Build history of the part. All positions in model axes, mm. Face numbers are marked on the shaded views. A direction names the side the tool comes from. Coordinates: 2 decimals unless noted, no trailing zeros. Loops run counter-clockwise (first coordinate to the right, second up) from the corner with the lowest first, then second, coordinate; pieces in that order, holes last. Notation, with made-up numbers: (67.25, -11.5) - (115.25, -11.5) arc R5 cw to (115.25, -4.5) - close; hole circle Ø8 at (71, 41). An arc over 180 degrees is marked (long way). One line per item, written item: value.
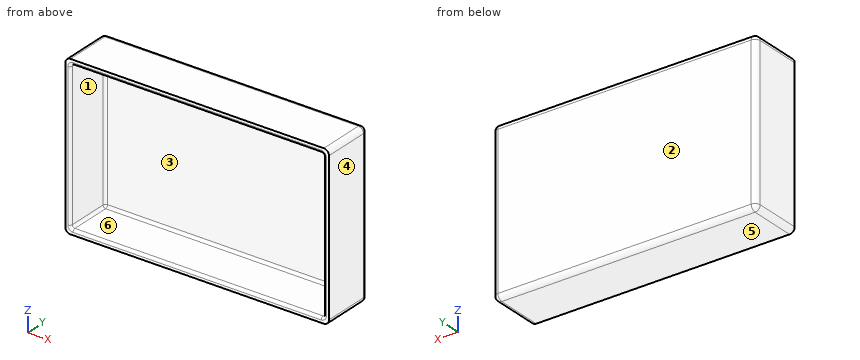
```python
from build123d import *

# Parameters (mm, degrees)
BOSS_EXTRUDE1_DEPTH = 20
FILLET1_R           = 2
SHELL1_START        = -49
SHELL1_OUTLINE_W    = 18
SHELL1_OUTLINE_H    = 58
SHELL1_DEPTH        = 98
FILLET2_R           = 1


# Read off the part's stored shape, not the designer's step: Shell1
with BuildPart() as part:
    # Sketch1 → Boss-Extrude1 (new body)
    with BuildSketch(Plane(origin=(0, 0, 0), x_dir=(1, 0, 0), z_dir=(0, 1, 0))):
        with BuildLine():
            Line((-49, -31), (49, -31))
            ThreePointArc((49, -31), (50.414213562, -30.414213562), (51, -29))
            Line((51, -29), (51, 29))
            ThreePointArc((51, 29), (50.414213562, 30.414213562), (49, 31))
            Line((49, 31), (-49, 31))
            ThreePointArc((-49, 31), (-50.414213562, 30.414213562), (-51, 29))
            Line((-51, 29), (-51, -29))
            ThreePointArc((-51, -29), (-50.414213562, -30.414213562), (-49, -31))
        make_face()
    extrude(amount=BOSS_EXTRUDE1_DEPTH)

    # Fillet1
    fillet1_edges = [part.edges().sort_by_distance(p)[0] for p in [
        (50.414213562, 20, -30.414213562),
        (0, 20, -31),
        (-50.414213562, 20, -30.414213562),
        (-51, 20, 0),
        (-50.414213562, 20, 30.414213562),
        (0, 20, 31),
        (50.414213562, 20, 30.414213562),
        (51, 20, 0),
    ]]
    fillet(fillet1_edges, radius=FILLET1_R)

    # Shell1 outline → Shell1 (cut)
    with BuildSketch(Plane.YZ.offset(SHELL1_START)):
        with Locations((9, 0)):
            Rectangle(SHELL1_OUTLINE_W, SHELL1_OUTLINE_H)
    extrude(amount=SHELL1_DEPTH, mode=Mode.SUBTRACT)

    # Fillet2
    fillet2_edges = [part.edges().sort_by_distance(p)[0] for p in [
        (49, 9, 29),
        (49, 0, 0),
        (0, 18, -29),
        (49, 9, -29),
        (0, 0, -29),
        (-49, 18, 0),
        (-49, 9, -29),
        (-49, 0, 0),
        (0, 18, 29),
        (-49, 9, 29),
        (0, 0, 29),
        (49, 18, 0),
    ]]
    fillet(fillet2_edges, radius=FILLET2_R)


solid = part.part
```
Item 1: Cut at A-A, the plane y = 13.5. Write the cut outline in (x, z).
Check result:
outline: (-51, -29) arc R2 ccw to (-49, -31) - (49, -31) arc R2 ccw to (51, -29) - (51, 29) arc R2 ccw to (49, 31) - (-49, 31) arc R2 ccw to (-51, 29) - close; hole (-49, -28) arc R1 ccw to (-48, -29) - (48, -29) arc R1 ccw to (49, -28) - (49, 28) arc R1 ccw to (48, 29) - (-48, 29) arc R1 ccw to (-49, 28) - close
Item 2: Tool access for the marked faces 1 and 2: list every direction of +Z, -Z, +X, -X, +Y, -Y with a clear straight run to the whole face (end or side of a thin tool).
Check result:
face 1: -Y
face 2: +Z, -Z, +X, -X, +Y
Item 3: Drop a flat-ended pin along its axis: P1, Ø2, axis at x = 3, z = 23, coming from the -Y side. Give the stop position or say it passes through.
Check result:
P1: stops at y = 18
Item 4: Pull direction X, two halves, no side cores. Call the marked faces 3, 4, 5 and 6: released by +X, released by -X, zero draft, split by the parting line, or undercut.
Check result:
face 3: undercut
face 4: released by +X
face 5: zero draft
face 6: undercut
Item 5: Cut at C-C, the plane z = 1. Write the cut outline in (x, y), then the cut area to 3 significant figures.
Check result:
outline: (-51, 0) - (-50, 0) arc R1 ccw to (-49, 1) - (-49, 17) arc R1 cw to (-48, 18) - (48, 18) arc R1 cw to (49, 17) - (49, 1) arc R1 ccw to (50, 0) - (51, 0) - (51, 18) arc R2 ccw to (49, 20) - (-49, 20) arc R2 ccw to (-51, 18) - close
area: 274 mm^2
Item 6: Cut at B-B, the plane x = 35. Write the cut outline in (y, z).
Check result:
outline: (0, -31) - (18, -31) arc R2 ccw to (20, -29) - (20, 29) arc R2 ccw to (18, 31) - (0, 31) - (0, 30) arc R1 ccw to (1, 29) - (17, 29) arc R1 cw to (18, 28) - (18, -28) arc R1 cw to (17, -29) - (1, -29) arc R1 ccw to (0, -30) - close
Item 7: Probe probe 1 along X at (y, z) = (5.25, 14); probe 2 along Z at (x, y) = (47, 10.5); probe 3 along Y at (x, z) = (42.5, 2). List the from-to ranges inside material, lowest first. Write a range as from..to.
Check result:
probe 1: x = -51..-49, 49..51
probe 2: z = -31..-29, 29..31
probe 3: y = 18..20
